```python
from build123d import *

# Parameters (mm, degrees)
SKETCH1_W              = 50
SKETCH1_H              = 300
BOSS_EXTRUDE1_DEPTH    = 3.175
CUT_EXTRUDE1_DEPTH     = 6.35
SKETCH3_R              = 5
SKETCH3_R_2            = 4.82
SKETCH3_R_3            = 1.025
CUT_EXTRUDE2_DEPTH     = 6.35
SKETCH4_R              = 3.175
SKETCH4_W              = 25
SKETCH4_H              = 100
CUT_EXTRUDE3_DEPTH     = 6.35
M2_5_CLEARANCE_HOLE1_D = 2.9


with BuildPart() as part:
    # Sketch1 → Boss-Extrude1 (new body)
    with BuildSketch(Plane(origin=(0, 0, 0), x_dir=(1, 0, 0), z_dir=(0, 1, 0))):
        with Locations((25, -150)):
            Rectangle(SKETCH1_W, SKETCH1_H)
    extrude(amount=BOSS_EXTRUDE1_DEPTH)

    # Sketch2 → Cut-Extrude1 (cut)
    with BuildSketch(Plane(origin=(0, 3.175, 0), x_dir=(1, 0, 0), z_dir=(0, 1, 0))):
        with BuildLine():
            ThreePointArc((25, 0), (42.67766953, -7.32233047), (50, -25))
            Line((50, -25), (50, 0))
            Line((50, 0), (25, 0))
        make_face()
        with BuildLine():
            Line((0, 0), (0, -25))
            ThreePointArc((0, -25), (7.32233047, -7.32233047), (25, 0))
            Line((25, 0), (0, 0))
        make_face()
        with BuildLine():
            Line((50, -300), (50, -275))
            ThreePointArc((50, -275), (42.67766953, -292.67766953), (25, -300))
            Line((25, -300), (50, -300))
        make_face()
        with BuildLine():
            ThreePointArc((25, -300), (7.32233047, -292.67766953), (0, -275))
            Line((0, -275), (0, -300))
            Line((0, -300), (25, -300))
        make_face()
    extrude(amount=-CUT_EXTRUDE1_DEPTH, mode=Mode.SUBTRACT)

    # Sketch3 → Cut-Extrude2 (cut)
    with BuildSketch(Plane(origin=(0, 3.175, 0), x_dir=(1, 0, 0), z_dir=(0, 1, 0))):
        with Locations(Location((25, -25, 0), (0, 0, 270))):
            Circle(SKETCH3_R)
        with Locations(Location((25, -275, 0), (0, 0, 270))):
            Circle(SKETCH3_R_2)
        with Locations(Location((25, -14, 0), (0, 0, 270))):
            Circle(SKETCH3_R_3)
        with Locations(Location((14, -25, 0), (0, 0, 270))):
            Circle(SKETCH3_R_3)
        with Locations(Location((25, -36, 0), (0, 0, 270))):
            Circle(SKETCH3_R_3)
        with Locations(Location((36, -25, 0), (0, 0, 270))):
            Circle(SKETCH3_R_3)
    extrude(amount=-CUT_EXTRUDE2_DEPTH, mode=Mode.SUBTRACT)

    # Sketch4 → Cut-Extrude3 (cut)
    with BuildSketch(Plane(origin=(0, 3.175, 0), x_dir=(1, 0, 0), z_dir=(0, 1, 0))):
        with Locations(Location((12.5, -80, 0), (0, 0, 270))):
            Circle(SKETCH4_R)
        with Locations(Location((12.5, -220, 0), (0, 0, 270))):
            Circle(SKETCH4_R)
        with Locations(Location((37.5, -220, 0), (0, 0, 270))):
            Circle(SKETCH4_R)
        with Locations(Location((37.5, -80, 0), (0, 0, 270))):
            Circle(SKETCH4_R)
        with Locations((25, -150)):
            Rectangle(SKETCH4_W, SKETCH4_H)
    extrude(amount=-CUT_EXTRUDE3_DEPTH, mode=Mode.SUBTRACT)

    # M2.5 Clearance Hole1 (through all)
    with Locations(Plane(origin=(0, 3.175, 0), x_dir=(1, 0, 0), z_dir=(0, 1, 0))):
        with Locations((14, -25), (25, -14), (36, -25), (25, -36)):
            Hole(M2_5_CLEARANCE_HOLE1_D / 2)


solid = part.part
```
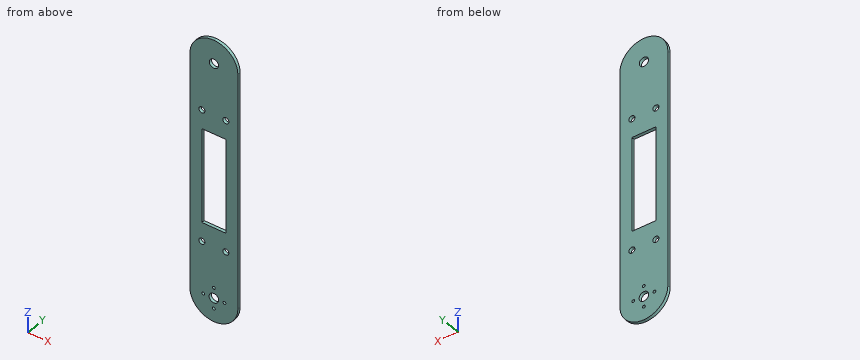
Work out the finished part from the listing and answer in its coordinate system (mm). Give positions to 0.01 mm unless a question says otherwise; leave off trailing zeros. Order: outer loops, then holes, each group sorted by start corner. A loop starts at its lowest first (then second) coordinate and runs counter-clockwise, first axis right, second up.
1. Section B-B, the plane y = 2.5 is taken. Give the number of separate pieces and of enclosed holes in the cut face, and give its area (3 significant figures).
Result sheet:
separate pieces: 1
enclosed holes: 11
area: 11,700 mm2
2. Each of these flat-tipped pins is pushed along its axis until it touches: P1, Ø1, axis at x = 21, y = 1, coming from the +Z side; P2, Ø5, axis at x = 37.5, z = 220, coming from the +Y side. Where does it stop, or does it pass through?
Result sheet:
P1: stops at z = 299.75
P2: passes through
3. Straight lines are drawn through the part: L1, parallel to X at y = 1.35, z = 25; L2, parallel to X at y = 1.45, z = 80 (3 decimals); L3, parallel to X at y = 0.5, z = 36. For each, find the intervals that lie inside material, in ascending order.
Result sheet:
L1: x = 0 to 12.55, 15.45 to 20, 30 to 34.55, 37.45 to 50
L2: x = 0 to 9.325, 15.675 to 34.325, 40.675 to 50
L3: x = 0 to 23.55, 26.45 to 50
4. Section A-A, the plane z = 116 is taken. Determine the outline of the cut face in (x, y) (3 decimals), and give its area (3 significant figures).
Result sheet:
outline: (0, 0) - (12.5, 0) - (12.5, 3.175) - (0, 3.175) - close; (37.5, 0) - (50, 0) - (50, 3.175) - (37.5, 3.175) - close
area: 79.4 mm2
